```python
from build123d import *

# Parameters (mm, degrees)
SKETCH_R        = 1.6
SKETCH_R_2      = 4.075
PAD_DEPTH       = 17.5
SKETCH001_R     = 4.075
POCKET_DEPTH    = 23.730537
SKETCH002_R     = 2.85
POCKET001_DEPTH = 2
POCKET002_DEPTH = 2.6
FILLET_R        = 2


with BuildPart() as part:
    # Sketch → Pad (new body)
    with BuildSketch(Plane.XY):
        with BuildLine():
            ThreePointArc((-7.5, 10.679537), (0, -13.05), (7.5, 10.679537))
            Line((-7.5, 10.679537), (7.5, 10.679537))
        make_face()
        with Locations((0, 7.377268)):
            Circle(SKETCH_R, mode=Mode.SUBTRACT)
        with Locations((0, -7.377268)):
            Circle(SKETCH_R, mode=Mode.SUBTRACT)
        Circle(SKETCH_R_2, mode=Mode.SUBTRACT)
    extrude(amount=PAD_DEPTH)

    # Sketch001 (on Face2 of Pad) → Pocket (cut, through all)
    with BuildSketch(Plane(origin=(0, 10.679537, 0), x_dir=(-1, 0, 0), z_dir=(0, 1, 0))):
        with Locations((0, 8.75)):
            Circle(SKETCH001_R)
    extrude(amount=-POCKET_DEPTH, mode=Mode.SUBTRACT)

    # Sketch002 (on Face3 of Pocket) → Pocket001 (cut)
    with BuildSketch(Plane(origin=(0, 0, 0), x_dir=(1, 0, 0), z_dir=(0, 0, -1))):
        with Locations((0, 7.377268)):
            Circle(SKETCH002_R)
        with Locations((0, -7.377268)):
            Circle(SKETCH002_R)
    extrude(amount=-POCKET001_DEPTH, mode=Mode.SUBTRACT)

    # Sketch003 (on Face4 of Pocket001) → Pocket002 (cut)
    with BuildSketch(Plane.XY.offset(17.5)):
        Polygon((1.616581, 10.177268), (-1.616581, 10.177268), (-3.233162, 7.377268), (-1.616581, 4.577268), (1.616581, 4.577268), (3.233162, 7.377268), align=None)
        Polygon((3.233162, -7.377268), (1.616581, -4.577268), (-1.616581, -4.577268), (-3.233162, -7.377268), (-1.616581, -10.177268), (1.616581, -10.177268), align=None)
    extrude(amount=-POCKET002_DEPTH, mode=Mode.SUBTRACT)

    # Fillet
    fillet_edges = [part.edges().sort_by_distance(p)[0] for p in [
        (0, -13.05, 0),
        (0, -13.05, 17.5),
    ]]
    fillet(fillet_edges, radius=FILLET_R)


solid = part.part
```
Design review of the part built by this model. Coordinates are the model's own, in mm. A direction names the side the tool comes from. Give positions to 0.01 mm unless a question says otherwise; leave off trailing zeros. Order: outer loops, then holes, each group sorted by start corner. A loop starts at its lowest first (then second) coordinate and runs counter-clockwise, first axis right, second up. Notation, with made-up numbers: (33, 62) - (87, 62) arc R24 cw to (87, 85) - close; hole circle Ø10 at (49.5, 86). An arc over 180 degrees is marked (long way). Use a Markdown table: item, result. Add a question column.
(1) Wall thickness on probe 1 along Y at (x, z) = (0, 13.8) (3 decimals); probe 2 along X at (y, z) = (0, 6.75) (3 decimals); probe 3 along X at (y, z) = (1.75, 13.5): over which ranges is each line inside the solid? List them lowest first. Write a range as [from, to].
(2) Mouldability with a two-part tool opening along Z and no side actions: class faces 1 (the face through (1, 9, 14.9)), 2 (the face through (4.07, 6.6, 8.93)), 3 (the face through (-3.003, 2.754, 3.342)), 4 (the face through (-2.191, -7.885, 12.186)) as +Z half, -Z half, draft (parallel to the pull), parting line (faces both ways), or undercut.
(3) Add section B-B on z = 13.5. Give the boundary of the cut face in (x, y) (3 decimals).
(4) Add section C-C on z = 5.75. Give the boundary of the cut face in (x, y) (3 decimals), then the cut area to 3 significant figures.
(5) Machinability: for faces 5 (the face through (-1.6, -7.3, 3.5)), 6 (the face through (-0.618, -4.595, 0.986)), 7 (the face through (2.436, 8.758, 16.218)), which of the approach directions +Z, -Z, +X, -X, +Y, -Y give a long, thin tool a straight path to every point of the face, cutting with its end or side? Answer none if there is none.
(6) Clearance check with flat-ended pins moving along their axes: P1, Ø4.5, axis at x = 0, y = -7.38, coming from the +Z side; P2, Ø4, axis at y = 8, z = 5.5, coming from the -X side; P3, Ø1.5, axis at x = -7, z = 8, coming from the -Y side. State where each tip first meets the part, or that it passes through.
(7) Add section A-A on z = 9.5. Give the boundary of the cut face in (x, y) (3 decimals).
Report:
| question | item | result |
|---|---|---|
| 1 | probe 1 | y = [-13.05, -8.977], [-5.777, -4.075], [4.075, 5.777], [8.977, 10.68] |
| 1 | probe 2 | x = [-13.05, -4.075], [4.075, 13.05] |
| 1 | probe 3 | x = [-12.93, -3.68], [3.68, 12.93] |
| 2 | face 1 | +Z half |
| 2 | face 2 | undercut |
| 2 | face 3 | draft |
| 2 | face 4 | undercut |
| 3 | outline | (-7.5, 10.68) arc R13.05 ccw (long way) to (7.5, 10.68) - close; hole circle Ø8.15 at (0, 0); hole circle Ø3.2 at (0, -7.377); hole circle Ø3.2 at (0, 7.377) |
| 4 | outline | (-7.5, 10.68) arc R13.05 ccw to (-2.758, -12.755) - (-2.758, -3) arc R4.075 cw to (-2.758, 3) - (-2.758, 10.68) - close; (2.758, -12.755) arc R13.05 ccw to (7.5, 10.68) - (2.758, 10.68) - (2.758, 3) arc R4.075 cw to (2.758, -3) - close |
| 4 | area | 370 mm² |
| 5 | face 5 | +Z, -Z |
| 5 | face 6 | -Z |
| 5 | face 7 | +Z |
| 6 | P1 | stops at z = 14.9 |
| 6 | P2 | stops at x = -11.59 |
| 6 | P3 | stops at y = -11.46 |
| 7 | outline | (-7.5, 10.68) arc R13.05 ccw to (-4.005, -12.42) - (-4.005, -0.75) arc R4.075 cw to (-4.005, 0.75) - (-4.005, 10.68) - close; (4.005, -12.42) arc R13.05 ccw to (7.5, 10.68) - (4.005, 10.68) - (4.005, 0.75) arc R4.075 cw to (4.005, -0.75) - close |
